from build123d import *

# Parameters (mm, degrees)
SZKIC2_R                    = 3.5
SZKIC2_R_2                  = 1.7
SZKIC2_R_3                  = 1.5
DODANIE_WYCI_GNI_CIE1_DEPTH = 5
SZKIC2_3_R                  = 3.5
SZKIC2_3_R_2                = 1.5
DODANIE_WYCI_GNI_CIE2_DEPTH = 3
WYTNIJ_WYCI_GNI_CIE1_DEPTH  = 6
SZYK_KO_OWY1_COUNT          = 4
ZAOKR_GLENIE1_R             = 4
SZKIC5_R                    = 3
WYTNIJ_WYCI_GNI_CIE3_DEPTH  = 3.5


with BuildPart() as part:
    # Szkic2 → Dodanie-wyci_gni_cie1 (new body)
    with BuildSketch(Plane(origin=(0, 0, 0), x_dir=(1, 0, 0), z_dir=(0, 1, 0))):
        with BuildLine():
            ThreePointArc((-23, -27), (-25.828427125, -25.828427125), (-27, -23))
            Line((-27, -23), (-27, 23))
            ThreePointArc((-27, 23), (-25.828427125, 25.828427125), (-23, 27))
            Line((-23, 27), (23, 27))
            ThreePointArc((23, 27), (25.828427125, 25.828427125), (27, 23))
            Line((27, 23), (27, -23))
            ThreePointArc((27, -23), (25.828427125, -25.828427125), (23, -27))
            Line((23, -27), (-23, -27))
        make_face()
        with Locations((15.695, -15.695)):
            Circle(SZKIC2_R, mode=Mode.SUBTRACT)
        with Locations((-15.695, -15.695)):
            Circle(SZKIC2_R, mode=Mode.SUBTRACT)
        with Locations((15.695, 15.695)):
            Circle(SZKIC2_R, mode=Mode.SUBTRACT)
        with Locations((-15.695, 15.695)):
            Circle(SZKIC2_R, mode=Mode.SUBTRACT)
        with Locations((-22.625, -22.625)):
            Circle(SZKIC2_R_2, mode=Mode.SUBTRACT)
        with Locations((22.625, -22.625)):
            Circle(SZKIC2_R_2, mode=Mode.SUBTRACT)
        with Locations((22.625, 22.625)):
            Circle(SZKIC2_R_2, mode=Mode.SUBTRACT)
        with Locations((-22.625, 22.625)):
            Circle(SZKIC2_R_2, mode=Mode.SUBTRACT)
        with Locations((15.695, 15.695)):
            Circle(SZKIC2_R)
        with Locations((15.695, 15.695)):
            Circle(SZKIC2_R_3, mode=Mode.SUBTRACT)
        with Locations((-15.695, 15.695)):
            Circle(SZKIC2_R)
        with Locations((-15.695, 15.695)):
            Circle(SZKIC2_R_3, mode=Mode.SUBTRACT)
        with Locations((15.695, -15.695)):
            Circle(SZKIC2_R)
        with Locations((15.695, -15.695)):
            Circle(SZKIC2_R_3, mode=Mode.SUBTRACT)
        with Locations((-15.695, -15.695)):
            Circle(SZKIC2_R)
        with Locations((-15.695, -15.695)):
            Circle(SZKIC2_R_3, mode=Mode.SUBTRACT)
    extrude(amount=-DODANIE_WYCI_GNI_CIE1_DEPTH)

    # Szkic2_3 → Dodanie-wyci_gni_cie2 (add)
    with BuildSketch(Plane(origin=(0, 0, 0), x_dir=(1, 0, 0), z_dir=(0, 1, 0))):
        with Locations((-15.695, 15.695)):
            Circle(SZKIC2_3_R)
        with Locations((-15.695, 15.695)):
            Circle(SZKIC2_3_R_2, mode=Mode.SUBTRACT)
        with Locations((15.695, 15.695)):
            Circle(SZKIC2_3_R)
        with Locations((15.695, 15.695)):
            Circle(SZKIC2_3_R_2, mode=Mode.SUBTRACT)
        with Locations((-15.695, -15.695)):
            Circle(SZKIC2_3_R)
        with Locations((-15.695, -15.695)):
            Circle(SZKIC2_3_R_2, mode=Mode.SUBTRACT)
        with Locations((15.695, -15.695)):
            Circle(SZKIC2_3_R)
        with Locations((15.695, -15.695)):
            Circle(SZKIC2_3_R_2, mode=Mode.SUBTRACT)
    extrude(amount=DODANIE_WYCI_GNI_CIE2_DEPTH)

    # Szkic3 → Wytnij-wyci_gni_cie1 (cut, through all)
    with BuildSketch(Plane(origin=(0, 0, 0), x_dir=(1, 0, 0), z_dir=(0, 1, 0))):
        Polygon((-7, -14), (7, -14), (20, -27), (-20, -27), align=None)
    wytnij_wyci_gni_cie1 = extrude(amount=-WYTNIJ_WYCI_GNI_CIE1_DEPTH, mode=Mode.SUBTRACT)

    # Szyk ko_owy1: Wytnij-wyci_gni_cie1 ×4 about axis
    szyk_ko_owy1_axis = Axis((0, 0, 0), (0, 1, 0))
    for i in range(1, SZYK_KO_OWY1_COUNT):
        add(wytnij_wyci_gni_cie1.rotate(szyk_ko_owy1_axis, i * 360 / SZYK_KO_OWY1_COUNT), mode=Mode.SUBTRACT)

    # Zaokr_glenie1
    zaokr_glenie1_edges = [part.edges().sort_by_distance(p)[0] for p in [
        (-7, -2.5, -14),
        (-20, -2.5, -27),
        (20, -2.5, -27),
        (7, -2.5, -14),
        (-14, -2.5, 7),
        (-27, -2.5, 20),
        (-27, -2.5, -20),
        (-14, -2.5, -7),
        (14, -2.5, -7),
        (27, -2.5, -20),
        (27, -2.5, 20),
        (14, -2.5, 7),
        (7, -2.5, 14),
        (20, -2.5, 27),
        (-20, -2.5, 27),
        (-7, -2.5, 14),
    ]]
    fillet(zaokr_glenie1_edges, radius=ZAOKR_GLENIE1_R)

    # Szkic5 → Wytnij-wyci_gni_cie3 (cut)
    with BuildSketch(Plane(origin=(0, 0, 0), x_dir=(1, 0, 0), z_dir=(0, 1, 0))):
        with Locations((-22.625, -22.625)):
            Circle(SZKIC5_R)
        with Locations((-22.625, 22.625)):
            Circle(SZKIC5_R)
        with Locations((22.625, 22.625)):
            Circle(SZKIC5_R)
        with Locations((22.625, -22.625)):
            Circle(SZKIC5_R)
    extrude(amount=-WYTNIJ_WYCI_GNI_CIE3_DEPTH, mode=Mode.SUBTRACT)


solid = part.part
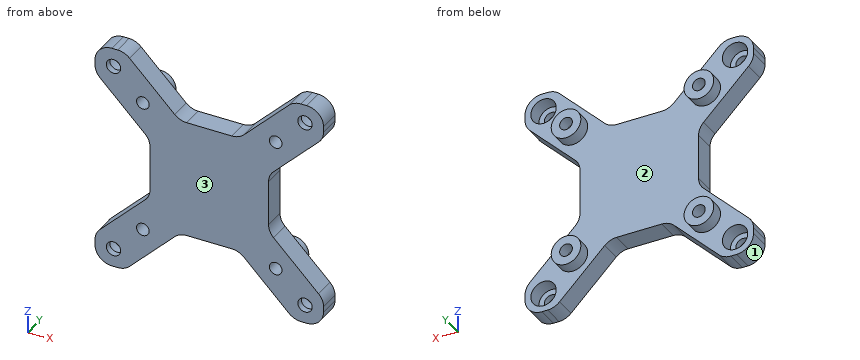
Input: part model. Units: mm. Frame: model coordinates. Face numbers are marked on the shaded views. Round coordinates to 2 decimals unless told otherwise and drop trailing zeros. Loops run counter-clockwise (first coordinate to the right, second up) from the corner with the lowest first, then second, coordinate; pieces in that order, holes last. Notation, with made-up numbers: (-25, 23) -> (-15, 23) arc R6 cw to (-15, 34) -> close; hole circle Ø10 at (-37, 51). An arc over 180 degrees is marked (long way). Answer as a JSON object with one key per item and string values. Group by question number.
1) Section query C-C on x = -13. Output: boundary loops of the cut face in (y, z).
2) Section query A-A on y = 1.75. Output: boundary loops of the cut face in (x, z) (3 decimals), plus the area to 3 significant figures.
3) Draft query along Z for the marked faces 1, 2 and 3. Return one class per face: +Z half, -Z half, draft (parallel to the pull), parting line (faces both ways), or undercut.
4) Ray query, L1, parallel to Z at x = -22, y = -1.25; L2, parallel to Z at x = 16.5, y = -2; L3, parallel to X at y = -2.75, z = -20.5. Return the intervals inside material, ascending.
5) Pin query (flat end, axial travel): pin 1 (2.5 mm diameter, centred on x = 15.695, z = 15.695, fed in from +Y); pin 2 (3 mm diameter, centred on x = -22, z = -23.5, fed in from +Y); pin 3 (7 mm diameter, centred on x = -22.625, z = -22.625, fed in from -Y); pin 4 (8 mm diameter, centred on x = -22.625, z = 22.625, fed in from +Y). Return the tip coordinate at first contact, or that it passes through.
6) Section query D-D on y = -1.5. State how many separate pieces and enclosed holes the cut face has, plus the area to 3 significant figures.
7) Section query B-B on z = -16.5. Output: boundary loops of the cut face in (x, y), plus the area to 3 significant figures.
Reply:
{
 "1": {"outline": "(-5, -20) -> (0, -20) -> (0, -17.93) -> (3, -17.93) -> (3, -13.46) -> (0, -13.46) -> (0, 13.46) -> (3, 13.46) -> (3, 17.93) -> (0, 17.93) -> (0, 20) -> (-5, 20) -> close"},
 "2": {"outline": "circle Ø7 at (-15.695, -15.695); circle Ø7 at (-15.695, 15.695); circle Ø7 at (15.695, -15.695); circle Ø7 at (15.695, 15.695); hole circle Ø3 at (-15.695, -15.695); hole circle Ø3 at (-15.695, 15.695); hole circle Ø3 at (15.695, -15.695); hole circle Ø3 at (15.695, 15.695)", "area": "126 mm2"},
 "3": {"face 1": "-Z half", "face 2": "undercut", "face 3": "draft"},
 "4": {"L1": "z = -27 to -25.56, -19.69 to -15, 15 to 19.69, 25.56 to 27", "L2": "z = -23.5 to -16.96, -14.43 to -9.5, 9.5 to 14.43, 16.96 to 23.5", "L3": "x = -26.83 to -24.74, -20.51 to -13.5, 13.5 to 20.51, 24.74 to 26.83"},
 "5": {"pin 1": "passes through", "pin 2": "stops at y = -3.5", "pin 3": "stops at y = -5", "pin 4": "stops at y = 0"},
 "6": {"separate pieces": "1", "enclosed holes": "8", "area": "1,360 mm2"},
 "7": {"outline": "(-23.5, -5) -> (-16.96, -5) -> (-16.96, 3) -> (-19.1, 3) -> (-19.1, 0) -> (-23.5, 0) -> close; (-14.43, -5) -> (-9.5, -5) -> (-9.5, 0) -> (-12.29, 0) -> (-12.29, 3) -> (-14.43, 3) -> close; (9.5, -5) -> (14.43, -5) -> (14.43, 3) -> (12.29, 3) -> (12.29, 0) -> (9.5, 0) -> close; (16.96, -5) -> (23.5, -5) -> (23.5, 0) -> (19.1, 0) -> (19.1, 3) -> (16.96, 3) -> close", "area": "140 mm2"}
}
